The drawing under review shows one solid part. Ordinate dimensions are in mm from its lowest x, y, z. A direction names the side the tool comes from. Round coordinates to 2 decimals unless told otherwise and drop trailing zeros. Order: outer loops, then holes, each group sorted by start corner. A loop starts at its lowest first (then second) coordinate and runs counter-clockwise, first axis right, second up. Notation, with made-up numbers: (60.25, 17) - (102.25, 17) arc R13 cw to (102.25, 22) - close; hole circle Ø3 at (73.5, -36.5). An arc over 180 degrees is marked (long way). One line per question, with ' | ' between items.
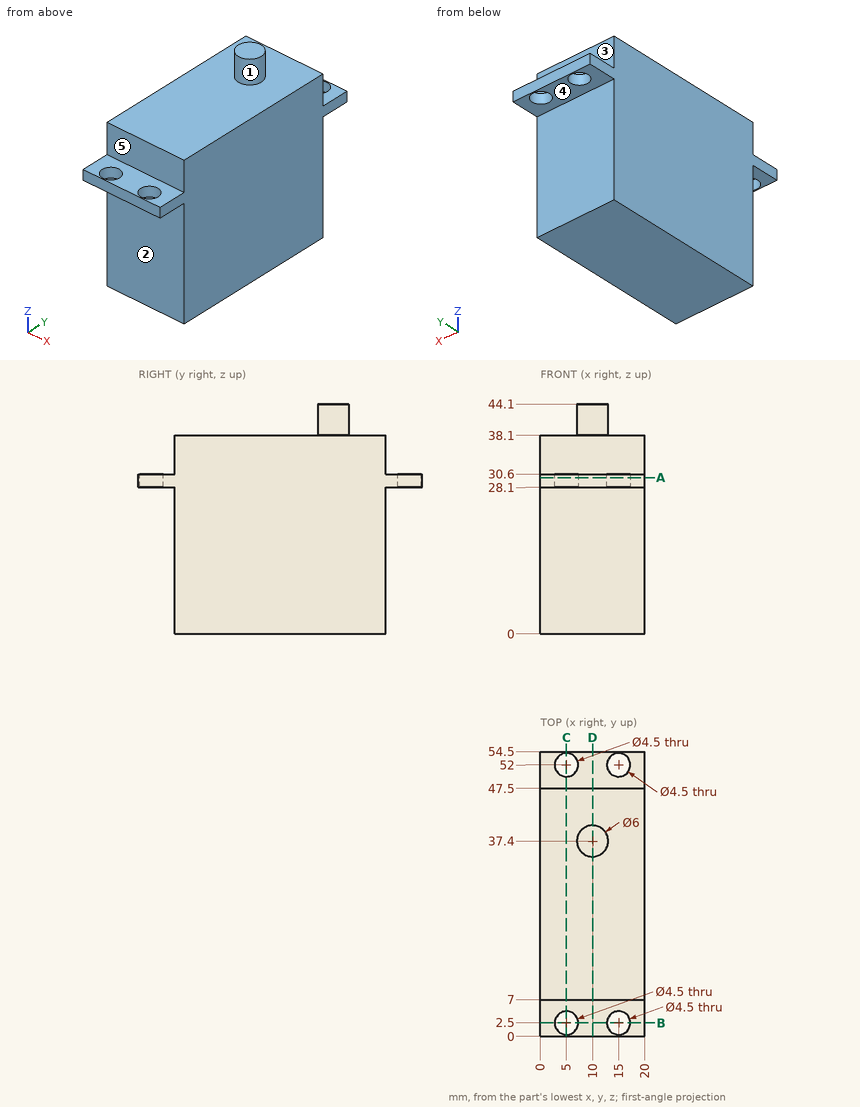
(1) For probe 1 along Y at (x, z) = (15, 29.75); probe 2 along Z at (x, y) = (14.5, 12.5); probe 3 along Y at (x, z) = (17.75, 15.5), list the stretches that pass through material, from the lowest coordinate up. Write a range as [from, to].
Output values:
probe 1: [0, 0.25], [4.75, 49.75], [54.25, 54.5] | probe 2: [0, 38.1] | probe 3: [7, 47.5]
(2) We need section A-A on z = 30. State the section outline as (x, y) points.
Output values:
outline: (0, 0) - (20, 0) - (20, 54.5) - (0, 54.5) - close; hole circle Ø4.5 at (5, 2.5); hole circle Ø4.5 at (5, 52); hole circle Ø4.5 at (15, 2.5); hole circle Ø4.5 at (15, 52)
(3) We need section D-D on x = 10. State the section outline as (y, z) points, plus the area to 3 significant figures.
Output values:
outline: (0, 28.1) - (7, 28.1) - (7, 0) - (47.5, 0) - (47.5, 28.1) - (54.5, 28.1) - (54.5, 30.6) - (47.5, 30.6) - (47.5, 38.1) - (40.4, 38.1) - (40.4, 44.1) - (34.4, 44.1) - (34.4, 38.1) - (7, 38.1) - (7, 30.6) - (0, 30.6) - close | area: 1,610 mm^2
(4) For the marked faces 1, 2, 3, 4 and 5, list the 3-axis set-ups (+Z, -Z, +X, -X, +Y, -Y) from which the entire face can be reached by the end or side of a thin tool; tool diameter is ignored.
Output values:
face 1: +Z | face 2: -Z, +X, -X, -Y | face 3: +Z, +X, -X, +Y | face 4: -Z, +X, -X, +Y | face 5: +Z, +X, -X, -Y
(5) Insertion check: pin 1 (1.5 mm diameter, centred on x = 7, z = 22, fed in from +Y); pin 2 (1 mm diameter, centred on x = 10.5, z = 17.5, fed in from -Y); pin 3 (5.5 mm diameter, centred on x = 12, y = 4, fed in from -Z); pin 4 (7.5 mm diameter, centred on x = 11.5, y = 50, fed in from -Z). Each pin has a flat end and moves straight along its axis. Give the tip position at first contact, or say it passes through.
Output values:
pin 1: y = 47.5 | pin 2: y = 7 | pin 3: z = 28.1 | pin 4: z = 0
(6) We need section B-B on y = 2.5. State the section outline as (x, z) points, plus the area to 3 significant figures.
Output values:
outline: (0, 28.1) - (2.75, 28.1) - (2.75, 30.6) - (0, 30.6) - close; (7.25, 28.1) - (12.75, 28.1) - (12.75, 30.6) - (7.25, 30.6) - close; (17.25, 28.1) - (20, 28.1) - (20, 30.6) - (17.25, 30.6) - close | area: 27.5 mm^2
(7) We need section C-C on x = 5. State the section outline as (y, z) points.
Output values:
outline: (0, 28.1) - (0.25, 28.1) - (0.25, 30.6) - (0, 30.6) - close; (4.75, 28.1) - (7, 28.1) - (7, 0) - (47.5, 0) - (47.5, 28.1) - (49.75, 28.1) - (49.75, 30.6) - (47.5, 30.6) - (47.5, 38.1) - (7, 38.1) - (7, 30.6) - (4.75, 30.6) - close; (54.25, 28.1) - (54.5, 28.1) - (54.5, 30.6) - (54.25, 30.6) - close
